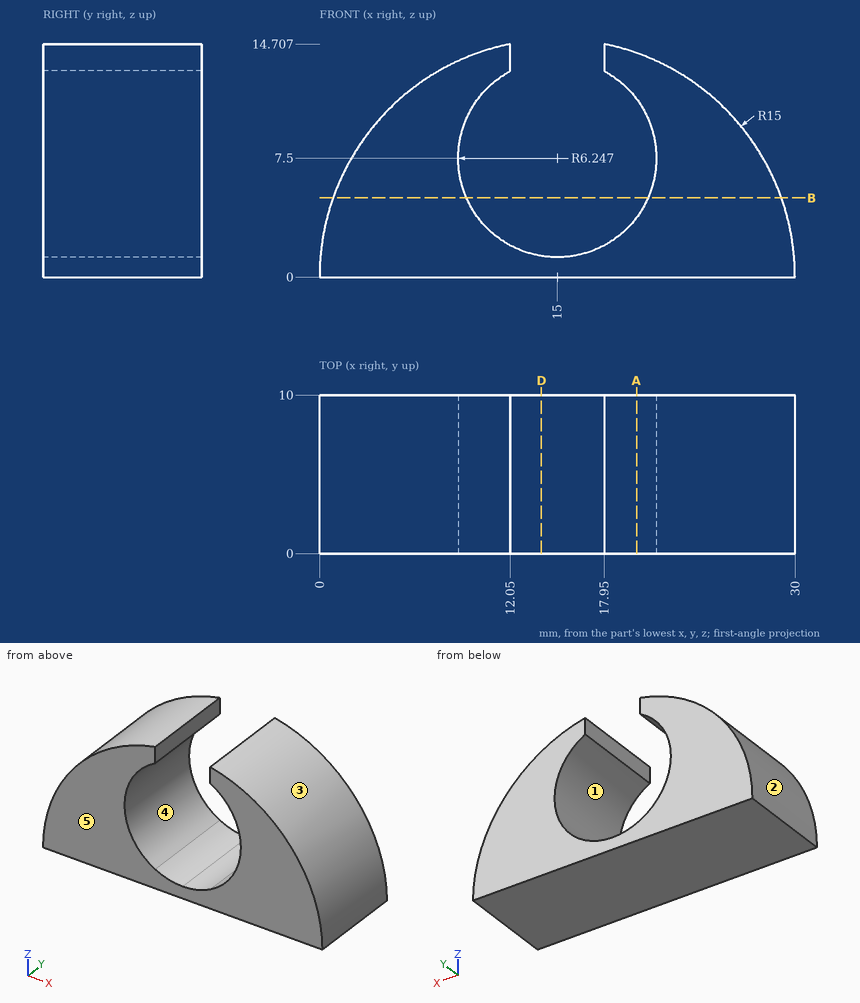
Study the drawing (mm; zero at the part's minimum x, y, z) and answer. A direction names the side the tool comes from. Coordinates: 2 decimals unless noted, no trailing zeros. Write each loop counter-clockwise with the first axis right and the second up, starting at its lowest first coordinate (ties: lowest second). Pieces come first, ordered by that corner, then holes. Notation, with made-up numbers: (15, 2) - (67, 2) arc R24 ccw to (67, 17) - close; hole circle Ø5 at (-5.5, 16.25). An arc over 180 degrees is marked (long way). Answer as a JSON object with one key per item and string values. Group by question number.
1. A cutting plane is placed at D-D (x = 14). Determine the outline of the cut face in (y, z).
2. Each of these flat-tipped pins is pushed along its axis until it touches: P1, Ø1.4, axis at y = 6, z = 13.5, coming from the +X side; P2, Ø3, axis at x = 26, z = 13, coming from the +Y side; P3, Ø3, axis at x = 18.5, z = 3.5, coming from the +Y side; P4, Ø0.5, axis at y = 5, z = 14, coming from the -X side (1 decimal). Where does it stop, or does it pass through?
3. Which of the six approach directions +Z, -Z, +X, -X, +Y, -Y give full straight-line access (tool end or side, diameter ignored) to the marked faces 1 and 2?
4. A cutting plane is placed at A-A (x = 20). Determine the outline of the cut face in (y, z) (1 decimal).
5. A cutting plane is placed at B-B (z = 5). Determine the outline of the cut face in (x, y) (1 decimal).
6. The mould has two halves that part along Z. Classify the marked faces 3, 4 and 5: +Z half, -Z half, draft (parallel to the pull), parting line (faces both ways), or undercut.
7. Consider L1, parallel to X at y = 0.5, z = 2.25 (1 decimal); L2, parallel to X at y = 3.75, z = 7 (1 decimal); L3, parallel to Z at x = 11.5, y = 7.5 (1 decimal). Determine where each line is inside the solid, lowest interval first. Write a range as [from, to].
Worked out:
{
 "1": {"outline": "(0, 0) - (10, 0) - (10, 1.33) - (0, 1.33) - close"},
 "2": {"P1": "stops at x = 22.82", "P2": "passes through", "P3": "stops at y = 10", "P4": "stops at x = 9"},
 "3": {"face 1": "+Y, -Y", "face 2": "+Z, -X, +Y, -Y"},
 "4": {"outline": "(0, 0) - (10, 0) - (10, 3.8) - (0, 3.8) - close; (0, 11.2) - (10, 11.2) - (10, 14.1) - (0, 14.1) - close"},
 "5": {"outline": "(0.9, 0) - (9.3, 0) - (9.3, 10) - (0.9, 10) - close; (20.7, 0) - (29.1, 0) - (29.1, 10) - (20.7, 10) - close"},
 "6": {"face 3": "+Z half", "face 4": "undercut", "face 5": "draft"},
 "7": {"L1": "x = [0.2, 11.6], [18.4, 29.8]", "L2": "x = [1.7, 8.8], [21.2, 28.3]", "L3": "z = [0, 2.3], [12.7, 14.6]"}
}
